The listing builds one solid part. Answer for the finished solid, in the listing's coordinates (mm). Face numbers are marked on the shaded views. A direction names the side the tool comes from. Give positions to 0.01 mm unless a question says otherwise; leave off trailing zeros. Loops run counter-clockwise (first coordinate to the right, second up) from the corner with the lowest first, then second, coordinate; pieces in that order, holes last. Notation, with made-up numbers: M 18,-10.75 L 72,-10.75 A24 cw 72,7.25 Z; hole C 25.25,4.25 d1. An arc over 180 degrees is marked long. Use one line per item in the form item = value. Start each with the question number.
1. Straight lines are drawn through the part: line 1 (Y direction, x = 30, z = 1.8); line 2 (X direction, y = 14, z = 1.3); line 3 (X direction, y = 37, z = 1.5). For each, find the intervals that lie inside material, in ascending order. Write a range as from..to.
2. The part is cut by section A-A (y = 16.5). Write down the section's boundary in (x, z).
3. The mould has two halves that part along X. Classify the marked faces 4, 5 and 6: released by +X, released by -X, zero draft, split by the parting line, or undercut.
4. Each of these flat-tipped pins is pushed along its axis until it touches: pin 1 Ø1.2 at (y, z) = (3, 2.5) entering from +X; pin 2 Ø2 at (x, z) = (40.5, 3) entering from -Y; pin 3 Ø2.5 at (x, y) = (30, 35.63) entering from -Z; pin 4 Ø1 at (x, z) = (17, 3) entering from +Y. Where does it stop, or does it pass through?
5. The part is cut by section C-C (y = 35). Write down the section's boundary in (x, z).
6. The part is cut by section B-B (x = 22.5). Write down the section's boundary in (y, z).
7. The part is cut by section D-D (z = 1.15). Give the number of separate pieces and of enclosed holes in the cut face, and give its area (3 significant figures).
8. For the marked faces 1, 2 and 3, determine the directions among +Z, -Z, +X, -X, +Y, -Y from which every point of the face is accessible in a straight line to the end or side of a thin tool.
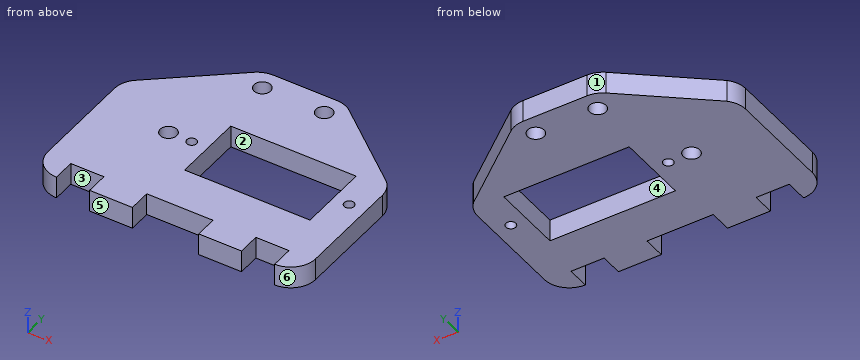
from build123d import *

# Parameters (mm, degrees)
SKETCH1_R           = 1.5
SKETCH1_R_2         = 0.9
SKETCH1_W           = 22.7
SKETCH1_H           = 12.9
BOSS_EXTRUDE1_DEPTH = 4


with BuildPart() as part:
    # Sketch1 → Boss-Extrude1 (new body)
    with BuildSketch(Plane.XY):
        with BuildLine():
            Line((48.50000085, 4.660421271), (48.50000085, 23.29646024))
            ThreePointArc((48.50000085, 23.29646024), (48.157458746, 25.018535686), (47.181981365, 26.478440755))
            Line((47.181981365, 26.478440755), (32.877904779, 38.147339677))
            ThreePointArc((32.877904779, 38.147339677), (31.543145465, 38.899591757), (30.033366148, 39.160421271))
            Line((30.033366148, 39.160421271), (18.466635551, 39.160421271))
            ThreePointArc((18.466635551, 39.160421271), (16.956856234, 38.899591757), (15.62209692, 38.147339677))
            Line((15.62209692, 38.147339677), (1.318020334, 26.478440755))
            ThreePointArc((1.318020334, 26.478440755), (0.342542953, 25.018535686), (8.5e-07, 23.29646024))
            Line((8.5e-07, 23.29646024), (8.5e-07, 4.660421271))
            ThreePointArc((8.5e-07, 4.660421271), (1.318020334, 1.478440755), (4.50000085, 0.160421271))
            Line((4.50000085, 0.160421271), (4.50000085, 4.160421271))
            Line((4.50000085, 4.160421271), (10.50000085, 4.160421271))
            Line((10.50000085, 4.160421271), (10.50000085, 0.160421271))
            Line((10.50000085, 0.160421271), (18.25000085, 0.160421271))
            Line((18.25000085, 0.160421271), (18.25000085, 4.160421271))
            Line((18.25000085, 4.160421271), (30.25000085, 4.160421271))
            Line((30.25000085, 4.160421271), (30.25000085, 0.160421271))
            Line((30.25000085, 0.160421271), (38.00000085, 0.160421271))
            Line((38.00000085, 0.160421271), (38.00000085, 4.160421271))
            Line((38.00000085, 4.160421271), (44.00000085, 4.160421271))
            Line((44.00000085, 4.160421271), (44.00000085, 0.160421271))
            ThreePointArc((44.00000085, 0.160421271), (47.181981365, 1.478440755), (48.50000085, 4.660421271))
        make_face()
        with Locations((12.80000085, 18.660421271)):
            Circle(SKETCH1_R, mode=Mode.SUBTRACT)
        with Locations((18.80000085, 35.630421271)):
            Circle(SKETCH1_R, mode=Mode.SUBTRACT)
        with Locations((30.00000085, 35.630421271)):
            Circle(SKETCH1_R, mode=Mode.SUBTRACT)
        with Locations((17.00000085, 18.660421271)):
            Circle(SKETCH1_R_2, mode=Mode.SUBTRACT)
        with Locations((45.50000085, 18.660421271)):
            Circle(SKETCH1_R_2, mode=Mode.SUBTRACT)
        with Locations((31.25000085, 18.660421271)):
            Rectangle(SKETCH1_W, SKETCH1_H, mode=Mode.SUBTRACT)
    extrude(amount=BOSS_EXTRUDE1_DEPTH)


solid = part.part
Derived:
q1.line_1 = 4.16..12.21, 25.11..34.13, 37.13..39.16
q1.line_2 = 0..19.9, 42.6..48.5
q1.line_3 = 14.22..18.19, 19.41..29.39, 30.61..34.28
q2.outline = M 0,0 L 19.9,0 L 19.9,4 L 0,4 Z; M 42.6,0 L 48.5,0 L 48.5,4 L 42.6,4 Z
q3.face_4 = undercut
q3.face_5 = zero draft
q3.face_6 = released by +X
q4.pin_1 = 48.37
q4.pin_2 = 4.16
q4.pin_3 = through
q4.pin_4 = 39.06
q5.outline = M 11.76,0 L 17.44,0 L 17.44,4 L 11.76,4 Z; M 20.16,0 L 28.64,0 L 28.64,4 L 20.16,4 Z; M 31.36,0 L 36.74,0 L 36.74,4 L 31.36,4 Z
q6.outline = M 4.16,0 L 12.21,0 L 12.21,4 L 4.16,4 Z; M 25.11,0 L 39.16,0 L 39.16,4 L 25.11,4 Z
q7.separate_pieces = 1
q7.enclosed_holes = 6
q7.area = 1,230 mm2
q8.face_1 = +Z, -Z, -X, +Y
q8.face_2 = +Z, -Z
q8.face_3 = +Z, -Z, -Y
